```python
from build123d import *

# Parameters (mm, degrees)
F1_DEPTH  = 25.4
F0_W      = 47.117
F0_H      = 14.859
F2_DEPTH  = 1.27
F4_DEPTH  = 1.27
F5_R      = 1.905
F6_DEPTH  = 1.27
F7_R      = 1.905
F8_DEPTH  = 1.27
F10_DEPTH = 63.5


with BuildPart() as f1:
    # F0 (on Front) → F1 (new body)
    with BuildSketch(Plane.XZ):
        with BuildLine():
            ThreePointArc((-58.928, 0), (-29.464, -2.286), (0, 0))
            Line((0, 0), (0, 16.891))
            Line((0, 16.891), (-5.9055, 16.891))
            Line((-5.9055, 16.891), (-5.9055, 2.032))
            Line((-5.9055, 2.032), (-53.0225, 2.032))
            Line((-53.0225, 2.032), (-53.0225, 16.891))
            Line((-53.0225, 16.891), (-58.928, 16.891))
            Line((-58.928, 16.891), (-58.928, 0))
        make_face()
    extrude(amount=F1_DEPTH)

    # F0 (on Front) → F2 (join)
    with BuildSketch(Plane.XZ):
        with Locations((-29.464, 9.4615)):
            Rectangle(F0_W, F0_H)
    extrude(amount=F2_DEPTH)

    # F3 (on face) → F4 (cut)
    with BuildSketch(Plane(origin=(0, 0, 0), x_dir=(-1, 0, 0), z_dir=(0, 1, 0))):
        with BuildLine():
            Line((58.928, 4.064), (0, 4.064))
            Line((0, 4.064), (0, 0))
            ThreePointArc((0, 0), (29.464, -2.286), (58.928, 0))
            Line((58.928, 0), (58.928, 4.064))
        make_face()
    extrude(amount=-F4_DEPTH, mode=Mode.SUBTRACT)

    # F5 (on face) → F6 (join)
    with BuildSketch(Plane(origin=(-5.9055, 0, 0), x_dir=(0, -1, 0), z_dir=(-1, 0, 0))):
        with Locations((7.874, 9.652)):
            Circle(F5_R)
    extrude(amount=F6_DEPTH)

    # F7 (on face) → F8 (join)
    with BuildSketch(Plane.YZ.offset(-53.0225)):
        with Locations((-7.874, 9.652)):
            Circle(F7_R)
    extrude(amount=F8_DEPTH)

    # F9 (on face) → F10 (cut)
    with BuildSketch(Plane.YZ):
        with BuildLine():
            ThreePointArc((-7.7890837565, 16.891), (-2.606552262, 14.45208016), (0, 9.3518009536))
            Line((0, 9.3518009536), (0, 16.891))
            Line((0, 16.891), (-7.7890837565, 16.891))
        make_face()
    extrude(amount=-F10_DEPTH, mode=Mode.SUBTRACT)


solid = f1.part
```
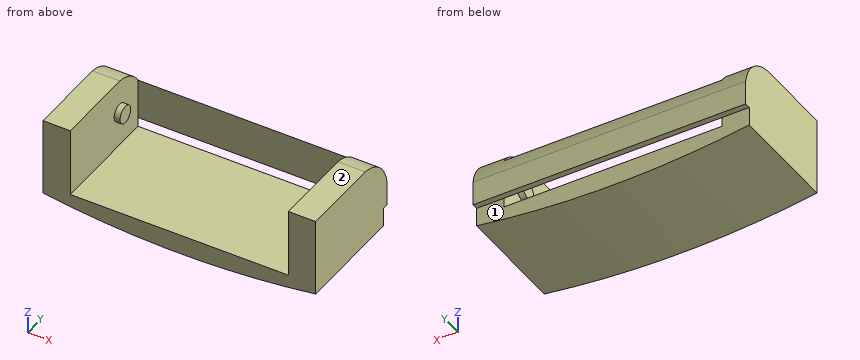
Part model, mm, in its own coordinate system. Face numbers are marked on the shaded views. A direction names the side the tool comes from. Give positions to 0.01 mm unless a question says otherwise; leave off trailing zeros. Loops run counter-clockwise (first coordinate to the right, second up) from the corner with the lowest first, then second, coordinate; pieces in that order, holes last. Notation, with made-up numbers: M -24.75,70 L 32.25,70 A18 ccw 32.25,88 Z; hole C 69.5,-5.5 d1. An arc over 180 degrees is marked long. Return JSON: item names as keys, results as strings.
1) 3-axis set-ups, long thin cutter, end or side, ignore diameter. For the marked faces 1 and 2: which of +Z, -Z, +X, -X, +Y, -Y reach the whole face in a straight line?
Calculated:
{"face 1": "-Z, +X, -X, +Y", "face 2": "+Z, +X, -X, +Y, -Y"}
2) Saw through at A-A, the plane x = -13. List the corners of the cut face in (y, z), then the cut area to 3 significant figures.
Calculated:
{"outline": "M -25.4,-1.58 L -1.27,-1.58 L -1.27,2.03 L -25.4,2.03 Z; M -1.27,4.06 L 0,4.06 L 0,9.35 A8.86 ccw -1.27,12.8 Z", "area": "96.4 mm2"}
3) Saw through at D-D, the plane y = -3.5. List the corners of the cut face in (x, z).
Calculated:
{"outline": "M -58.93,0 A191.02 ccw 0,0 L 0,15.21 L -5.91,15.21 L -5.91,2.03 L -53.02,2.03 L -53.02,15.21 L -58.93,15.21 Z"}
4) Flat gauge pins, fed straight in: pin 1 Ø3 at (x, z) = (-24, -0.5) entering from +Y; pin 2 Ø12 at (x, y) = (-10, -22) entering from -Z; pin 3 Ø7 at (x, z) = (-23.5, 7) entering from -Y. Where does each tip first touch, or does it go through?
Calculated:
{"pin 1": "stops at y = -1.27", "pin 2": "stops at z = -1.81", "pin 3": "stops at y = -1.27"}
5) Saw through at C-C, the plane y = -13. List the corners of the cut face in (x, z).
Calculated:
{"outline": "M -58.93,0 A191.02 ccw 0,0 L 0,16.89 L -5.91,16.89 L -5.91,2.03 L -53.02,2.03 L -53.02,16.89 L -58.93,16.89 Z"}
6) Drill centre lines: line 1 (X direction, y = -7, z = 8.5); line 2 (X direction, y = -23.5, z = 12.5); line 3 (Y direction, x = -15.5, z = 9). Where is each one in solid material? Low to high.
Calculated:
{"line 1": "x = -58.93 to -51.75, -7.18 to 0", "line 2": "x = -58.93 to -53.02, -5.91 to 0", "line 3": "y = -1.27 to 0"}
7) Saw through at B-B, the plane z = 15.25. List the corners of the cut face in (x, y), then the cut area to 3 significant figures.
Calculated:
{"outline": "M -58.93,-25.4 L -53.02,-25.4 L -53.02,-3.56 L -58.93,-3.56 Z; M -5.91,-25.4 L 0,-25.4 L 0,-3.56 L -5.91,-3.56 Z", "area": "258 mm2"}
